```python
from build123d import *

# Parameters (mm, degrees)
BOSS_EXTRUDE1_DEPTH      = 14.5
BOSS_EXTRUDE2_REACH      = 65.963
BOSS_EXTRUDE2_END_RADIUS = 26.5
SKETCH4_R                = 0.5
BOSS_EXTRUDE3_DEPTH      = 5
SKETCH6_R                = 2.5
BOSS_EXTRUDE4_DEPTH      = 19.5
SKETCH7_R                = 18
SKETCH7_R_2              = 2.5
CUT_EXTRUDE1_DEPTH       = 7
SKETCH8_R                = 1
CUT_EXTRUDE2_DEPTH       = 50.558046814
SKETCH9_R                = 1.5
CUT_EXTRUDE3_DEPTH       = 5


with BuildPart() as part:
    # Sketch1 → Boss-Extrude1 (new, symmetric)
    with BuildSketch(Plane.XY):
        with BuildLine():
            Line((-20, 20.885338651), (-20, -13.885338651))
            ThreePointArc((-20, -13.885338651), (0, -23), (20, -13.885338651))
            Line((20, -13.885338651), (20, 20.885338651))
            ThreePointArc((20, 20.885338651), (0, 30), (-20, 20.885338651))
        make_face()
    extrude(amount=BOSS_EXTRUDE1_DEPTH, both=True)

    # Boss-Extrude2: up to this cylinder (the profile starts outside it)
    boss_extrude2_end = Plane(origin=(0, 3.5, -3.065471), z_dir=(0, 0, -1)) * Cylinder(BOSS_EXTRUDE2_END_RADIUS, 185.926, mode=Mode.PRIVATE)
    # Sketch3 → Boss-Extrude2 (add, up to the surface)
    with BuildSketch(Plane(origin=(0, -29, 0), x_dir=(1, 0, 0), z_dir=(0, 1, 0)), mode=Mode.PRIVATE) as boss_extrude2_sk1:
        with BuildLine():
            Line((-11.658910532, 14.5), (2.658910532, 14.5))
            ThreePointArc((2.658910532, 14.5), (5.85802759, 10.496124943), (7, 5.5))
            Line((7, 5.5), (7, -7.5))
            Line((7, -7.5), (-16, -7.5))
            Line((-16, -7.5), (-16, 5.5))
            ThreePointArc((-16, 5.5), (-14.85802759, 10.496124943), (-11.658910532, 14.5))
        make_face()
    boss_extrude2_tool1 = extrude(boss_extrude2_sk1.sketch, amount=BOSS_EXTRUDE2_REACH, mode=Mode.PRIVATE) - boss_extrude2_end
    add(boss_extrude2_tool1.solids().sort_by_distance((-4.5, -29, -3.065471))[0])

    # Sketch4 → Boss-Extrude3 (add)
    with BuildSketch(Plane.XY.offset(7.5)):
        with Locations(Location((-11.5, -25, 0), (0, 0, 180))):
            Circle(SKETCH4_R)
        with Locations(Location((2.5, -25, 0), (0, 0, 180))):
            Circle(SKETCH4_R)
    extrude(amount=BOSS_EXTRUDE3_DEPTH)

    # Sketch6 → Boss-Extrude4 (add, symmetric)
    with BuildSketch(Plane.XY):
        Circle(SKETCH6_R)
    extrude(amount=BOSS_EXTRUDE4_DEPTH, both=True)

    # Sketch7 → Cut-Extrude1 (cut)
    with BuildSketch(Plane.XY.offset(14.5)):
        Circle(SKETCH7_R)
        Circle(SKETCH7_R_2, mode=Mode.SUBTRACT)
    extrude(amount=-CUT_EXTRUDE1_DEPTH, mode=Mode.SUBTRACT)

    # Sketch8 → Cut-Extrude2 (cut, through all)
    with BuildSketch(Plane.XY.offset(14.5)):
        with Locations((-15.5, 19.5)):
            Circle(SKETCH8_R)
        with Locations((15.5, 19.5)):
            Circle(SKETCH8_R)
        with Locations((15.5, -12.5)):
            Circle(SKETCH8_R)
        with Locations((-15.5, -12.5)):
            Circle(SKETCH8_R)
    extrude(amount=-CUT_EXTRUDE2_DEPTH, mode=Mode.SUBTRACT)

    # Sketch9 → Cut-Extrude3 (cut)
    with BuildSketch(Plane(origin=(20, 0, 0), x_dir=(0, 0, -1), z_dir=(1, 0, 0))):
        with Locations(Location((0, 11, 0), (0, 0, 90))):
            Circle(SKETCH9_R)
        with Locations(Location((0, -4, 0), (0, 0, 90))):
            Circle(SKETCH9_R)
    cut_extrude3 = extrude(amount=-CUT_EXTRUDE3_DEPTH, mode=Mode.SUBTRACT)

    # Mirror1: Cut-Extrude3 across plane
    add(cut_extrude3.mirror(Plane(origin=(0, 0, 0), x_dir=(0, 0, 1), z_dir=(1, 0, 0))), mode=Mode.SUBTRACT)


solid = part.part
```
Can you work these out from the model? Positions are in its coordinate system, mm. A direction names the side the tool comes from. Give positions to 0.01 mm unless a question says otherwise; leave off trailing zeros. Write each loop counter-clockwise with the first axis right and the second up, starting at its lowest first coordinate (ties: lowest second). Pieces come first, ordered by that corner, then holes. Notation, with made-up numbers: (3, 62.25) - (54, 62.25) arc R7 cw to (54, 70.25) - close; hole circle Ø3 at (-31, 2). An arc over 180 degrees is marked (long way). Write item = value, one per line. Start each with the question number.
1. On a 3-axis mill with a long thin cutter (end or side, diameter ignored), from which of +Z, -Z, +X, -X, +Y, -Y can I reach the whole of each face in a straight line? I mean faces 1 (the face through (7, -26, 1)), 2 (the face through (17.54, 9.5, 0.07)), 3 (the face through (-17.54, 9.5, 0.07)). Say none if no direction works.
2. Imagine slicing it at B-B (z = 3.5). Please give me the cut outline in (x, y), and give its area (3 significant figures).
3. Imagine slicing it at A-A (z = 10.5). Count the separate pieces of the cut face and the enclosed holes in it, and give its area (3 significant figures).
4. For pin 1 (5.5 mm diameter, centred on x = -6, y = -23, fed in from +Z); pin 2 (5.5 mm diameter, centred on y = -21.5, z = 0, fed in from -X); pin 3 (1.5 mm diameter, centred on y = 23.5, z = -15, fed in from +X), each with a flat end and sliding along its axis, tell me the tip position at first contact or that it passes through.
5. Imagine slicing it at D-D (x = 0). Please give me the cut outline in (y, z).
6. Thinking about a two-plate mould opening in X: for faces 4 (the face through (0, 0, 19.5)), 5 (the face through (-0.54, -2.44, 13.58)), 6 (the face through (15, -4, 0)), which applies, released by +X, released by -X, zero draft, split by the parting line, or undercut?
7. Imagine slicing it at C-C (y = -12.5). Please give me the cut outline in (x, z), and give its area (3 significant figures).
8. Please list where these lines run through material, in increasing order: line 1 (X direction, y = 19, z = 0); line 2 (Y direction, x = 15.5, z = -0.25); line 3 (Z direction, x = -16, y = 11).
Worked answers:
q1.face_1 = +Z, -Z, +X, -Y
q1.face_2 = +X
q1.face_3 = -X
q2.outline = (-20, -13.89) arc R26.5 ccw to (-16, -17.62) - (-16, -29) - (7, -29) - (7, -22.06) arc R26.5 ccw to (20, -13.89) - (20, 20.89) arc R26.5 ccw to (-20, 20.89) - close; hole circle Ø2 at (-15.5, -12.5); hole circle Ø2 at (-15.5, 19.5); hole circle Ø2 at (15.5, -12.5); hole circle Ø2 at (15.5, 19.5)
q2.area = 2,050 mm2
q3.separate_pieces = 4
q3.enclosed_holes = 5
q3.area = 887 mm2
q4.pin_1 = 14.5
q4.pin_2 = -16
q4.pin_3 = 18.01
q5.outline = (-29, -14.5) - (-2.5, -14.5) - (-2.5, -19.5) - (2.5, -19.5) - (2.5, -14.5) - (30, -14.5) - (30, 14.5) - (18, 14.5) - (18, 7.5) - (2.5, 7.5) - (2.5, 19.5) - (-2.5, 19.5) - (-2.5, 7.5) - (-18, 7.5) - (-18, 14.5) - (-23, 14.5) - (-23, 7.5) - (-29, 7.5) - close
q6.face_4 = zero draft
q6.face_5 = undercut
q6.face_6 = released by +X
q7.outline = (-20, -14.5) - (-16.5, -14.5) - (-16.5, 14.5) - (-20, 14.5) - close; (-14.5, -14.5) - (14.5, -14.5) - (14.5, 14.5) - (12.95, 14.5) - (12.95, 7.5) - (-12.95, 7.5) - (-12.95, 14.5) - (-14.5, 14.5) - close; (16.5, -14.5) - (20, -14.5) - (20, 14.5) - (16.5, 14.5) - close
q7.area = 863 mm2
q8.line_1 = -20 to -16.37, -14.63 to 14.63, 16.37 to 20
q8.line_2 = -17.99 to -13.5, -11.5 to -5.48, -2.52 to 9.52, 12.48 to 18.5, 20.5 to 24.99
q8.line_3 = -14.5 to -1.5, 1.5 to 14.5
